```python
from build123d import *

# Parameters (mm, degrees)
F1_DEPTH = 30
F3_D     = 3.3
F4_R     = 5


with BuildPart() as f1:
    # F0 (on Right) → F1 (new body)
    with BuildSketch(Plane.YZ):
        Polygon((-15.9727102009, 16.1656831887), (-15.9727102009, -3.8343168113), (-13.9727102009, -3.8343168113), (-13.9727102009, 15.1685199726), (1.2036300463, 26.6047126317), (0, 28.2019836518), align=None)
    extrude(amount=F1_DEPTH)

    # F3 (through all)
    with Locations(Plane(origin=(0, -13.554743317, 17.9877519272), x_dir=(1, 0, 0), z_dir=(0, -0.6018150232, 0.79863551))):
        with Locations((15, 6.9723774443)):
            Hole(F3_D / 2)

    # F4
    f4_edges = [f1.edges().sort_by_distance(p)[0] for p in [
        (15, -15.97271, 16.165683),
        (15, -13.97271, 15.16852),
    ]]
    fillet(f4_edges, radius=F4_R)


solid = f1.part
```
Model file for the job. Use its own axes, mm. A direction names the side the tool comes from. Give positions to 0.01 mm unless a question says otherwise; leave off trailing zeros. Write each loop counter-clockwise with the first axis right and the second up, starting at its lowest first coordinate (ties: lowest second). Pieces come first, ordered by that corner, then holes. Notation, with made-up numbers: M 30,67 L 71,67 A28 ccw 71,97 Z; hole C 78.25,44.25 d1. An arc over 180 degrees is marked long. Use a Markdown table: item, result.
1) Pin check, flat tips, straight feed: pin 1 (8 mm diameter, centred on x = 7.5, y = -4, fed in from -Z); pin 2 (2 mm diameter, centred on x = 6, z = 15, fed in from +Y); pin 3 (5 mm diameter, centred on x = 25, y = -9.5, fed in from +Z). Stop position of each tip, or through.
Responses:
| item | result |
|---|---|
| pin 1 | stops at z = 19.67 |
| pin 2 | stops at y = -12.71 |
| pin 3 | stops at z = 22.93 |
2) Pull direction Y, two halves, no side cores. Call faces 3 (the flat face through (14.79, 0.61, 27.39)), 4 (the cylindrical face through (13.476, -7.881, 20.994)), 5 (the flat face through (30, -14, 15)), 6 (the cylindrical face through (15.21, -15.462, 15.875)): +Y half, -Y half, draft (parallel to the pull), parting line (faces both ways), or undercut.
Responses:
| item | result |
|---|---|
| face 3 | +Y half |
| face 4 | undercut |
| face 5 | draft |
| face 6 | -Y half |
3) Cut at B-B (x = 21.25). List the corners of the cut face in (y, z), and give its area (3 significant figures).
Responses:
| item | result |
|---|---|
| outline | M -15.97,-3.83 L -13.97,-3.83 L -13.97,12.68 A5 cw -11.98,16.67 L 1.2,26.6 L 0,28.2 L -13.98,17.67 A5 ccw -15.97,13.67 Z |
| area | 78.0 mm2 |
4) Cut at D-D (y = -3.25). List the corners of the cut face in (x, z).
Responses:
| item | result |
|---|---|
| outline | M 0,23.25 L 30,23.25 L 30,25.75 L 0,25.75 Z |
5) Cut at A-A (x = 14). List the corners of the cut face in (y, z), and give its area (3 significant figures).
Responses:
| item | result |
|---|---|
| outline | M -15.97,-3.83 L -13.97,-3.83 L -13.97,12.68 A5 cw -11.98,16.67 L -7.83,19.8 L -9.03,21.39 L -13.98,17.67 A5 ccw -15.97,13.67 Z; M -6.94,22.97 L -5.73,21.38 L 1.2,26.6 L 0,28.2 Z |
| area | 72.8 mm2 |
6) Tool access for faces 1 (the flat face through (14.79, -5.34, 24.18)), 2 (the flat face through (15, -13.973, 4)): list every direction of +Z, -Z, +X, -X, +Y, -Y with a clear straight run to the whole face (end or side of a thin tool).
Responses:
| item | result |
|---|---|
| face 1 | +Z, +X, -X, -Y |
| face 2 | -Z, +X, -X, +Y |
7) Drill centre lines: line 1 (Y direction, x = 5, z = 3); line 2 (Z direction, x = 24, y = -8.5); line 3 (Z direction, x = 28.75, y = -5). Where is each one in solid material? Low to high. Write a range as from..to.
Responses:
| item | result |
|---|---|
| line 1 | y = -15.97..-13.97 |
| line 2 | z = 19.29..21.8 |
| line 3 | z = 21.93..24.43 |
8) Cut at C-C (z = 1.5). List the corners of the cut face in (x, y), and give its area (3 significant figures).
Responses:
| item | result |
|---|---|
| outline | M 0,-15.97 L 30,-15.97 L 30,-13.97 L 0,-13.97 Z |
| area | 60.0 mm2 |
